```python
from build123d import *

# Parameters (mm, degrees)
SKETCH1_W           = 76
SKETCH1_H           = 20
BOSS_EXTRUDE1_DEPTH = 6
SKETCH2_R           = 2.4
CUT_EXTRUDE1_DEPTH  = 6
FILLET1_R           = 2


with BuildPart() as part:
    # Sketch1 → Boss-Extrude1 (new body)
    with BuildSketch(Plane(origin=(0, 0, 0), x_dir=(1, 0, 0), z_dir=(0, 1, 0))):
        with Locations((38, 10)):
            Rectangle(SKETCH1_W, SKETCH1_H)
    extrude(amount=BOSS_EXTRUDE1_DEPTH)

    # Sketch2 → Cut-Extrude1 (cut)
    with BuildSketch(Plane(origin=(0, 6, 0), x_dir=(1, 0, 0), z_dir=(0, 1, 0))):
        with Locations((9.5, 10)):
            Circle(SKETCH2_R)
        with BuildLine():
            Line((71.5, 13.914396505), (71.5, 6.085603495))
            ThreePointArc((71.5, 6.085603495), (60.15, 10), (71.5, 13.914396505))
        make_face()
    extrude(amount=-CUT_EXTRUDE1_DEPTH, mode=Mode.SUBTRACT)

    # Fillet1
    fillet1_edges = [part.edges().sort_by_distance(p)[0] for p in [
        (76, 6, -10),
        (38, 6, -20),
        (0, 6, -10),
        (38, 0, -20),
        (76, 0, -10),
        (38, 0, 0),
        (0, 0, -10),
        (38, 6, 0),
        (0, 3, -20),
        (76, 3, -20),
        (76, 3, 0),
        (0, 3, 0),
    ]]
    fillet(fillet1_edges, radius=FILLET1_R)


solid = part.part
```
Part model, mm, in its own coordinate system. Round coordinates to 2 decimals unless told otherwise and drop trailing zeros. Order: outer loops, then holes, each group sorted by start corner. A loop starts at its lowest first (then second) coordinate and runs counter-clockwise, first axis right, second up. Notation, with made-up numbers: M 61,58 L 88,58 A34 ccw 88,95 Z; hole C 33,19.5 d1. An arc over 180 degrees is marked long. Answer in a Markdown table with one row per item. Add a question column.
Q1. Cut at C-C on x = 32. Give the cut face in (y, z).
Q2. Cut at B-B on z = -11.5. Give the cut face in (x, y).
Q3. Cut at A-A on x = 9.5. Give the cut face in (y, z).
Q4. Wall check: L1, parallel to Z at x = 9.5, y = 3.6; L2, parallel to Z at x = 66.5, y = 3.2; L3, parallel to X at y = 5.1, z = -10.75. Give the ranges that are in metal, low to high. Write a range as from..to.
Q5. Mould opens along Z. For faces 1 (the face through (29, 6, -10)), 2 (the face through (75.4, 3.01, -19.43)), 3 (the face through (60.154, 3.042, -9.78)) say: +Z half, -Z half, draft (parallel to the pull), parting line (faces both ways), or undercut.
Q6. Pin check, flat tips, straight feed: pin 1 (7.5 mm diameter, centred on x = 9.5, z = -10, fed in from -Y); pin 2 (1 mm diameter, centred on y = 1, z = -10.5, fed in from -X); pin 3 (7.5 mm diameter, centred on x = 66.5, z = -10, fed in from +Y). Stop position of each tip, or through.
Q7. Cut at D-D on y = 5.05. Give the cut face in (x, z).
Established:
| question | item | result |
|---|---|---|
| 1 | outline | M 0,-18 A2 ccw 2,-20 L 4,-20 A2 ccw 6,-18 L 6,-2 A2 ccw 4,0 L 2,0 A2 ccw 0,-2 Z |
| 2 | outline | M 0,2 A2 ccw 2,0 L 7.63,0 L 7.63,6 L 2,6 A2 ccw 0,4 Z; M 11.37,0 L 60.33,0 L 60.33,6 L 11.37,6 Z; M 71.5,0 L 74,0 A2 ccw 76,2 L 76,4 A2 ccw 74,6 L 71.5,6 Z |
| 3 | outline | M 0,-18 A2 ccw 2,-20 L 4,-20 A2 ccw 6,-18 L 6,-12.4 L 0,-12.4 Z; M 0,-7.6 L 6,-7.6 L 6,-2 A2 ccw 4,0 L 2,0 A2 ccw 0,-2 Z |
| 4 | L1 | z = -20..-12.4, -7.6..0 |
| 4 | L2 | z = -20..-16.35, -3.65..0 |
| 4 | L3 | x = 0.33..7.22, 11.78..60.19, 71.5..75.67 |
| 5 | face 1 | draft |
| 5 | face 2 | -Z half |
| 5 | face 3 | undercut |
| 6 | pin 1 | stops at y = 0 |
| 6 | pin 2 | stops at x = 0.06 |
| 6 | pin 3 | passes through |
| 7 | outline | M 0.3,-18 A1.7 ccw 2,-19.7 L 74,-19.7 A1.7 ccw 75.7,-18 L 75.7,-2 A1.7 ccw 74,-0.3 L 2,-0.3 A1.7 ccw 0.3,-2 Z; hole C 9.5,-10 d4.8; hole M 71.5,-13.91 L 71.5,-6.09 A6.35 ccw long Z |
